Geometry check sheet. Reference: the model listing, model coordinates, mm. Face numbers are marked on the shaded views. A direction names the side the tool comes from. Give positions to 0.01 mm unless a question says otherwise; leave off trailing zeros. Order: outer loops, then holes, each group sorted by start corner. A loop starts at its lowest first (then second) coordinate and runs counter-clockwise, first axis right, second up.
from build123d import *

# Parameters (mm, degrees)
BOSS_EXTRUDE1_DEPTH      = 0.3
BOSS_EXTRUDE2_DEPTH      = 3
BOSS_EXTRUDE2_DEPTH_BACK = 3
BOSS_EXTRUDE2_START      = -1.75
SKETCH2_W                = 0.3
SKETCH2_H                = 13.5
BOSS_EXTRUDE3_DEPTH      = 3
BOSS_EXTRUDE3_DEPTH_BACK = 3
BOSS_EXTRUDE3_START      = -1.75
CUT_EXTRUDE1_REACH       = 19.264
SKETCH4_R                = 0.75
CUT_EXTRUDE2_REACH       = 18.483
SKETCH7_W                = 0.3
SKETCH7_H                = 1.8
CUT_EXTRUDE3_DEPTH       = 1
BOSS_EXTRUDE4_DEPTH      = 1
BOSS_EXTRUDE5_DEPTH      = 1
FILLET1_R                = 0.5


with BuildPart() as part:
    # Sketch1 → Boss-Extrude1 (new body)
    with BuildSketch(Plane(origin=(0, 0, 0), x_dir=(1, 0, 0), z_dir=(0, 1, 0))):
        Polygon((-2, 3), (2, 3), (2, -3), (-2, -3), (-2, -1.75), (-4.5, -1.75), (-4.5, 1.75), (-2, 1.75), align=None)
    extrude(amount=BOSS_EXTRUDE1_DEPTH)

    # Sketch2 → Boss-Extrude2 (add, two sides: drawn at the far end of the back side and taken through both)
    with BuildSketch(Plane.XY.offset(1.75).offset(BOSS_EXTRUDE2_START - BOSS_EXTRUDE2_DEPTH_BACK)):
        with Locations((-4.65, 6.75)):
            Rectangle(SKETCH2_W, SKETCH2_H)
    extrude(amount=BOSS_EXTRUDE2_DEPTH + BOSS_EXTRUDE2_DEPTH_BACK)

    # Sketch3 → Boss-Extrude3 (add, two sides: drawn at the far end of the back side and taken through both)
    with BuildSketch(Plane.XY.offset(1.75).offset(BOSS_EXTRUDE3_START - BOSS_EXTRUDE3_DEPTH_BACK)):
        with BuildLine():
            Line((-6.5, 13.554573958), (-8.505448086, 9.369290995))
            ThreePointArc((-8.505448086, 9.369290995), (-8.725435374, 8.737631794), (-8.8, 8.072930454))
            Line((-8.8, 8.072930454), (-8.8, 5.754573958))
            Line((-8.8, 5.754573958), (-8.5, 5.754573958))
            Line((-8.5, 5.754573958), (-8.5, 8.072930454))
            ThreePointArc((-8.5, 8.072930454), (-8.432891837, 8.67116166), (-8.234903278, 9.239654941))
            Line((-8.234903278, 9.239654941), (-6.224158485, 13.435991899))
            add(Edge.make_bspline(
                [(-4.8, 13.499999998), (-4.800000001, 13.60647764), (-4.810501359, 13.834290272), (-4.865595968, 14.168326182), (-4.985627931, 14.441197759), (-5.11401111, 14.537231122), (-5.274676327, 14.571482274), (-5.645213861, 14.387952807), (-6.003576613, 13.924542153), (-6.162685709, 13.596781364), (-6.224158485, 13.435991899)],
                knots=[0, 0, 0, 0, 0.062658964, 0.125317927, 0.250635855, 0.375953782, 0.50127171, 0.751907565, 0.877225492, 1.00254342, 1.00254342, 1.00254342, 1.00254342], degree=3))
            Line((-4.8, 13.499999998), (-4.5, 13.5))
            add(Edge.make_bspline(
                [(-4.5, 13.5), (-4.500000011, 15.507992756), (-5.926328545, 15.055080891), (-6.5, 13.554573958)],
                knots=[0, 0, 0, 0, 1, 1, 1, 1], degree=3))
        make_face()
    extrude(amount=BOSS_EXTRUDE3_DEPTH + BOSS_EXTRUDE3_DEPTH_BACK)

    # Sketch4 → Cut-Extrude1 (cut, up to next)
    with BuildSketch(Plane(origin=(0, 0.3, 0), x_dir=(1, 0, 0), z_dir=(0, 1, 0)), mode=Mode.PRIVATE) as cut_extrude1_sk1:
        with Locations(Location((0, 0, 0), (0, 0, 270))):
            Circle(SKETCH4_R)
    cut_extrude1_tool1 = extrude(cut_extrude1_sk1.sketch, amount=-CUT_EXTRUDE1_REACH, mode=Mode.PRIVATE) & part.part
    add(cut_extrude1_tool1.solids().sort_by_distance((0, 0.3, 0))[0], mode=Mode.SUBTRACT)

    # Sketch6 → Cut-Extrude2 (cut, up to next)
    with BuildSketch(Plane(origin=(-4.5, 0, 0), x_dir=(0, 0, -1), z_dir=(1, 0, 0)), mode=Mode.PRIVATE) as cut_extrude2_sk1:
        Polygon((1.75, 1.8), (1.75, 0.3), (1.75, 0), (3, 0), (3, 1.8), align=None)
    cut_extrude2_tool1 = extrude(cut_extrude2_sk1.sketch, amount=-CUT_EXTRUDE2_REACH, mode=Mode.PRIVATE) & part.part
    # Sketch6 → Cut-Extrude2 (cut, up to next)
    with BuildSketch(Plane(origin=(-4.5, 0, 0), x_dir=(0, 0, -1), z_dir=(1, 0, 0)), mode=Mode.PRIVATE) as cut_extrude2_sk2:
        Polygon((-1.75, 0.3), (-1.75, 1.8), (-3, 1.8), (-3, 0), (-1.75, 0), align=None)
    cut_extrude2_tool2 = extrude(cut_extrude2_sk2.sketch, amount=-CUT_EXTRUDE2_REACH, mode=Mode.PRIVATE) & part.part
    add(cut_extrude2_tool1.solids().sort_by_distance((-4.5, 0.9, -2.375))[0], mode=Mode.SUBTRACT)
    add(cut_extrude2_tool2.solids().sort_by_distance((-4.5, 0.9, 2.375))[0], mode=Mode.SUBTRACT)

    # Sketch7 → Cut-Extrude3 (cut)
    with BuildSketch(Plane.XY.offset(3)):
        with Locations((-4.65, 6.4)):
            Rectangle(SKETCH7_W, SKETCH7_H)
    cut_extrude3 = extrude(amount=-CUT_EXTRUDE3_DEPTH, mode=Mode.SUBTRACT)

    # Mirror1: Cut-Extrude3 across plane
    add(cut_extrude3.mirror(Plane.XY), mode=Mode.SUBTRACT)

    # Sketch8 → Boss-Extrude4 (add)
    with BuildSketch(Plane.XY.offset(3)):
        Polygon((-4.5, 5.5), (-4, 6.7), (-4, 7.3), (-4.3, 7.3), (-4.3, 6.7), (-4.8, 5.5), align=None)
    boss_extrude4 = extrude(amount=-BOSS_EXTRUDE4_DEPTH)

    # Mirror2: Boss-Extrude4 across plane
    add(boss_extrude4.mirror(Plane.XY))

    # Sketch9 → Boss-Extrude5 (add)
    with BuildSketch(Plane.XY.offset(3)):
        with BuildLine():
            Line((-4.8, 9.3), (-4.8, 10.3))
            ThreePointArc((-4.8, 10.3), (-5.007106781, 9.8), (-4.8, 9.3))
        make_face()
    boss_extrude5 = extrude(amount=-BOSS_EXTRUDE5_DEPTH)

    # Mirror4: Boss-Extrude5 across plane
    add(boss_extrude5.mirror(Plane.XY))

    # Fillet1
    fillet1_edges = [part.edges().sort_by_distance(p)[0] for p in [
        (-4.5, 0.3, 0),
        (-4.8, 0, 0),
    ]]
    fillet(fillet1_edges, radius=FILLET1_R)


solid = part.part
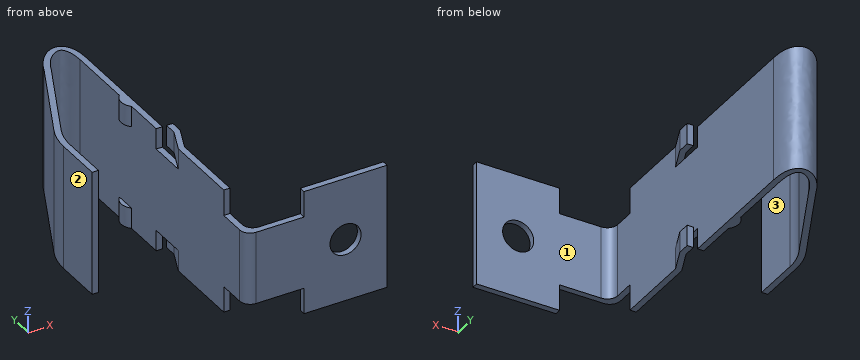
Item 1: Set-up check for the marked faces 1, 2 and 3: record each of +Z, -Z, +X, -X, +Y, -Y from which the full face is reachable in a straight line by a thin tool's end or side.
Reported:
face 1: +Z, -Z, +X, +Y
face 2: +Z, -Z, -X, +Y, -Y
face 3: +Z, -Z, -Y
Item 2: Sectioned sample at B-B (y = 12.5). Enter the section's corners in (x, z), and give its area (3 significant figures).
Reported:
outline: (-7.01, -3) - (-6.67, -3) - (-6.67, 3) - (-7.01, 3) - close; (-4.8, -3) - (-4.5, -3) - (-4.5, 3) - (-4.8, 3) - close
area: 3.80 mm2
Item 3: Scan lines: L1, parallel to X at y = 3.5, z = -0.5; L2, parallel to Y at x = 0, z = 1.75; L3, parallel to X at y = 10.25, z = 2.25. Record each from-to range of solid material in increasing order.
Reported:
L1: x = -4.8 to -4.5
L2: y = 0 to 0.3
L3: x = -8.08 to -7.75, -4.85 to -4.5
Item 4: Sectioned sample at C-C (z = 2.25). Give the number of separate pieces and of enclosed holes in the cut face, and give its area (3 significant figures).
Reported:
separate pieces: 3
enclosed holes: 0
area: 8.29 mm2
Item 5: Gauge pin test, flat ends, axial feed: pin 1 (0.9 mm diameter, centred on x = -3.5, y = 0.5, fed in from +Z); pin 2 (3 mm diameter, centred on x = -1, z = -1.5, fed in from +Y); pin 3 (1.9 mm diameter, centred on y = 6.5, z = -1, fed in from +X). Record the tip position at first contact, or that the pin passes through.
Reported:
pin 1: stops at z = 1.75
pin 2: stops at y = 0.3
pin 3: stops at x = -4.5
Item 6: Sectioned sample at A-A (x = 0). Enter the section's corners in (y, z).
Reported:
outline: (0, -3) - (0.3, -3) - (0.3, -0.75) - (0, -0.75) - close; (0, 0.75) - (0.3, 0.75) - (0.3, 3) - (0, 3) - close
Item 7: Sectioned sample at D-D (y = 3.25). Enter the section's corners in (x, z), and give its area (3 significant figures).
Reported:
outline: (-4.8, -3) - (-4.5, -3) - (-4.5, 3) - (-4.8, 3) - close
area: 1.80 mm2
